Input: dimensioned drawing with shaded views. Units: mm. Origin: part minimum x, y, z. A direction names the side the tool comes from. Coordinates: 2 decimals unless noted, no trailing zeros. Order: outer loops, then holes, each group sorted by start corner. A loop starts at its lowest first (then second) coordinate and runs counter-clockwise, first axis right, second up.
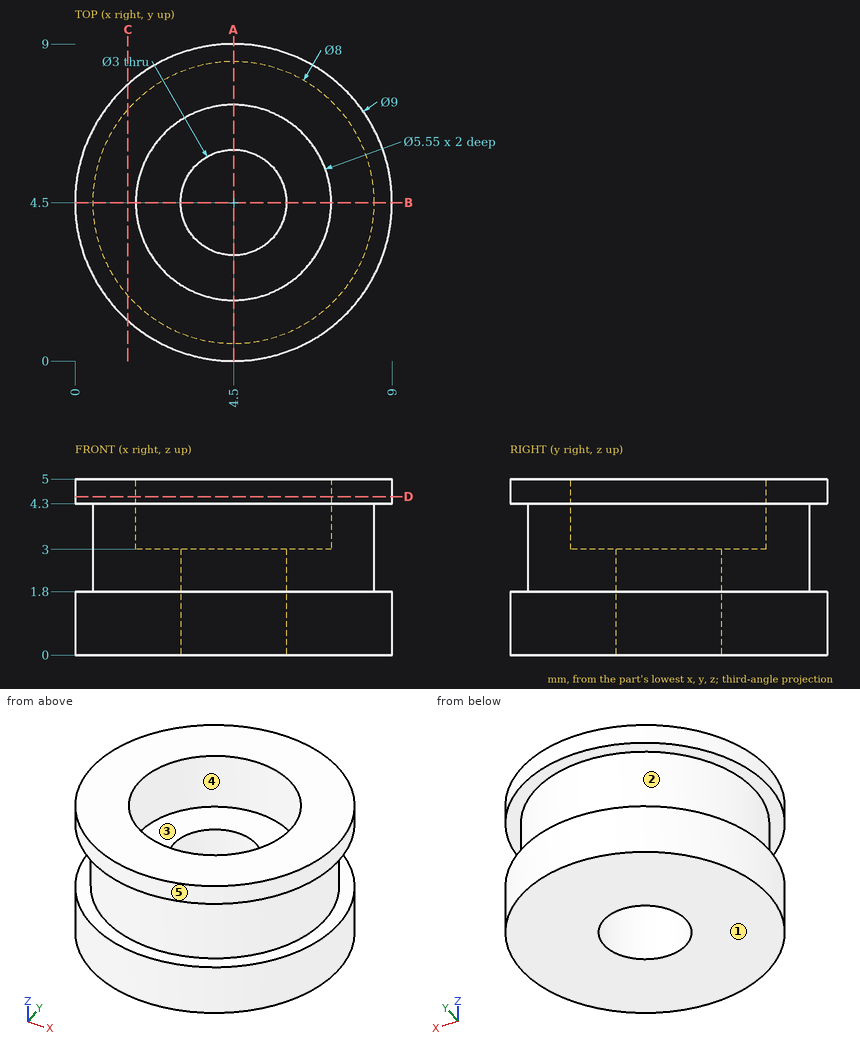
1. Section query A-A on x = 4.5. Return loops of the section in (y, z) (3 decimals), plus the area to 3 significant figures.
Findings:
outline: (0, 0) - (3, 0) - (3, 3) - (1.725, 3) - (1.725, 5) - (0, 5) - (0, 4.3) - (0.5, 4.3) - (0.5, 1.8) - (0, 1.8) - close; (6, 0) - (9, 0) - (9, 1.8) - (8.5, 1.8) - (8.5, 4.3) - (9, 4.3) - (9, 5) - (7.275, 5) - (7.275, 3) - (6, 3) - close
area: 22.4 mm2
2. Draft query along Y for the marked faces 1, 2 and 3. Return one class per face: released by +Y, released by -Y, zero draft, split by the parting line, or undercut.
Findings:
face 1: zero draft
face 2: split by the parting line
face 3: undercut
3. Section query C-C on x = 1.5. Return loops of the section in (y, z), plus the area to 3 significant figures.
Findings:
outline: (1.15, 0) - (7.85, 0) - (7.85, 1.8) - (7.15, 1.8) - (7.15, 4.3) - (7.85, 4.3) - (7.85, 5) - (1.15, 5) - (1.15, 4.3) - (1.85, 4.3) - (1.85, 1.8) - (1.15, 1.8) - close
area: 30.0 mm2
4. Section query D-D on z = 4.5. Return loops of the section in (x, y) (3 decimals).
Findings:
outline: circle Ø9 at (4.5, 4.5); hole circle Ø5.55 at (4.5, 4.5)
5. Ray query, line 1 (Z direction, x = 3.25, y = 8.5); line 2 (Y direction, x = 4.5, z = 4.6) (3 decimals); line 3 (Y direction, x = 4.5, z = 2.15). Return the intervals inside material, ascending.
Findings:
line 1: z = 0 to 1.8, 4.3 to 5
line 2: y = 0 to 1.725, 7.275 to 9
line 3: y = 0.5 to 3, 6 to 8.5
6. Access query for the marked faces 4 and 5. Directions: +Z, -Z, +X, -X, +Y, -Y. A direction counts if a zero-diameter tool reaches every point of the face in a straight line with its end or side. Return the directions, or none.
Findings:
face 4: +Z
face 5: +Z, -Z
7. Pin query (flat end, axial travel): P1, Ø5, axis at x = 4.5, y = 4.5, coming from the +Z side; P2, Ø2, axis at x = 2, z = 4, coming from the +Y side. Return the tip coordinate at first contact, or that it passes through.
Findings:
P1: stops at z = 3
P2: stops at y = 8.73
